The listing builds one solid part. Answer for the finished solid, in the listing's coordinates (mm). Face numbers are marked on the shaded views. Round coordinates to 2 decimals unless told otherwise and drop trailing zeros. Write each loop counter-clockwise with the first axis right and the second up, starting at its lowest first coordinate (ties: lowest second). Pieces come first, ordered by that corner, then holes.
Item 1: Find section D-D on x = 1.05. Give the vertices of the cut face in (y, z), then the cut area to 3 significant figures.
Item 2: Find section A-A on y = 0.45. Give the number of separate pieces and of enclosed holes in the cut face, then the cut area to 3 significant figures.
Item 3: Find the intervals of material crossed by probe 1 along Z at (x, y) = (-0.15, 2.2); probe 2 along Y at (x, z) = (-0.45, -6); probe 3 along X at (y, z) = (1.8, 1.5), in increasing order.
Item 4: Each of these flat-tipped pins is pushed along its axis until it touches: pin 1 (1.2 mm diameter, centred on x = 0, z = 0.5, fed in from +Y); pin 2 (1.5 mm diameter, centred on x = 1.5, y = 2.5, fed in from -Z); pin 3 (1 mm diameter, centred on y = 0.5, z = -1.5, fed in from +X). Where does it stop, or does it pass through?
Item 5: For a pull along X with two mould halves and no side action, classify the marked faces 1, 2, 3 and 4 as +X half, -X half, draft (parallel to the pull), parting line (faces both ways), or undercut.
Item 6: Find section B-B on z = 8.25. Give the vertices of the cut face in (x, y).
Autodesk Inventor part; units mm, degrees
ref_plane "YZ Plane" through (0, 0, 0) normal (1, 0, 0) x (0, 1, 0)
ref_plane "XZ Plane" through (0, 0, 0) normal (0, 1, 0) x (-1, 0, 0)
ref_plane "XY Plane" through (0, 0, 0) normal (0, 0, 1) x (1, 0, 0)
sketch "Sketch1" plane through (0, 0, 0) normal (0, 1, 0) x (-1, 0, 0)
  circle A0 centre (0, 0) radius 2.75
  circle A1 centre (0, 12) radius 1.5
  circle A2 centre (0, -12) radius 1.5
  line L0 (0, 12) -> (0, -12) construction
  line L1 (2.735, -0.2865) -> (1.4918, -12.1562)
  line L2 (-1.4918, 12.1563) -> (-2.735, 0.2865)
  line L3 (-1.4918, -12.1562) -> (-2.735, -0.2865)
  line L4 (1.4918, 12.1563) -> (2.735, 0.2865)
  dimension "d0" = 5.5
  dimension "d1" = 3
  dimension "d2" = 27
extrude "Extrusion1" add sketch "Sketch1" along normal blind 1
sketch "Sketch2" plane through (0, 1, 0) normal (0, 1, 0) x (1, 0, 0)
  circle A0 centre (0, 0) radius 2.75
  circle A1 centre (0, 0) radius 2
  dimension "d5" = 5.5
  dimension "d6" = 4
extrude "Extrusion2" add sketch "Sketch2" along normal blind 2
sketch "Sketch3" plane through (0, 0, 0) normal (0, -1, 0) x (1, 0, 0)
  line L0 (-1.4918, -12.1562) -> (-2.735, -0.2865)
  arc A0 (-1.4918, -12.1562) -> (1.4918, -12.1562) centre (0, -12) ccw
  line L1 (2.735, -0.2865) -> (1.4918, -12.1562)
  arc A1 (2.735, -0.2865) -> (2.735, 0.2865) centre (0, 0) ccw
  line L2 (1.4918, 12.1563) -> (2.735, 0.2865)
  arc A2 (1.4918, 12.1563) -> (-1.4918, 12.1563) centre (0, 12) ccw
  line L3 (-2.735, 0.2865) -> (-1.4918, 12.1563)
  arc A3 (-2.735, 0.2865) -> (-2.735, -0.2865) centre (0, 0) ccw
  circle A4 centre (0, -12) radius 0.5
  circle A5 centre (0, -10) radius 0.5
  circle A6 centre (0, -8) radius 0.5
  circle A7 centre (0, 8) radius 0.5
  circle A8 centre (0, 10) radius 0.5
  circle A9 centre (0, 12) radius 0.5
  dimension "d9" = 1
  dimension "d10" = 1
  dimension "d11" = 1
  dimension "d12" = 1
  dimension "d13" = 1
  dimension "d16" = 180
extrude "Extrusion3" cut sketch "Sketch3" against normal through all contours A4 | A5 | A6 | A7 | A8 | A9
properties part number "Dual Servo Attachment" material "ABS Plastic"
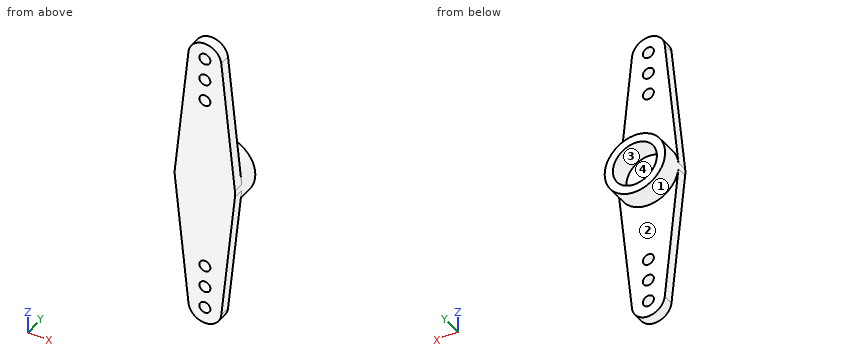
Check values:
1. outline: (0, -13.07) - (1, -13.07) - (1, -2.54) - (3, -2.54) - (3, -1.7) - (1, -1.7) - (1, 1.7) - (3, 1.7) - (3, 2.54) - (1, 2.54) - (1, 13.07) - (0, 13.07) - close
1. area: 29.5 mm2
2. separate pieces: 1
2. enclosed holes: 6
2. area: 105 mm2
3. probe 1: z = -2.75 to -1.99, 1.99 to 2.75
3. probe 2: y = 0 to 1
3. probe 3: x = -2.3 to -1.32, 1.32 to 2.3
4. pin 1: stops at y = 1
4. pin 2: stops at z = -2.65
4. pin 3: stops at x = 2.66
5. face 1: parting line
5. face 2: draft
5. face 3: undercut
5. face 4: undercut
6. outline: (-1.9, 0) - (-0.43, 0) - (-0.43, 1) - (-1.9, 1) - close; (0.43, 0) - (1.9, 0) - (1.9, 1) - (0.43, 1) - close
